Geometry check sheet. Reference: the model listing, model coordinates, mm. Coordinates: 2 decimals unless noted, no trailing zeros. Order: outer loops, then holes, each group sorted by start corner. A loop starts at its lowest first (then second) coordinate and runs counter-clockwise, first axis right, second up. Notation, with made-up numbers: (35.25, -34) -> (56.25, -34) arc R20 ccw to (56.25, -26) -> close; hole circle Ø7 at (20, 10.5). An arc over 180 degrees is marked (long way). Answer in a Markdown table with one row per item. Add a question column.
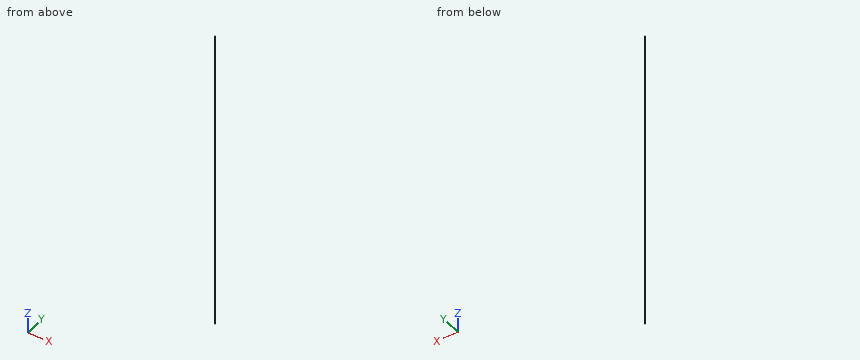
```python
from build123d import *

# Parameters (mm, degrees)
F0_R     = 4.7625
F1_DEPTH = 1295.4
F2_R     = 4.699
F3_DEPTH = 50.8
F5_SIZE  = 0.762


with BuildPart() as f1:
    # F0 (on Top) → F1 (new body, symmetric)
    with BuildSketch(Plane.XY):
        Circle(F0_R)
    extrude(amount=F1_DEPTH, both=True)

    # F2 (on face) → F3 (join)
    with BuildSketch(Plane.XY.offset(1295.4)):
        Circle(F2_R)
    extrude(amount=F3_DEPTH)

    # F4: F1 across plane


with BuildPart() as f1_1:
    add(f1.part)
    add(f1.part.mirror(Plane.XY))

    # F5
    f5_edges = [f1_1.edges().sort_by_distance(p)[0] for p in [
        (-4.699, 0, 1346.2),
        (-4.699, 0, -1346.2),
    ]]
    chamfer(f5_edges, length=F5_SIZE)


solid = f1_1.part
```
(1) Cross-section at A-A (z = 703). Enter the section's corners in (x, y) (1 decimal), plus the area to 3 significant figures.
(2) Go/stop test with flat-tipped pins: P1, Ø1, axis at y = -1, z = 203.5, coming from the +X side; P2, Ø5, axis at y = -1.5, z = 83, coming from the +X side; P3, Ø1.5, axis at x = -3.5, z = -978.5, coming from the +Y side; P4, Ø5, axis at y = -4, z = 15, coming from the +X side. Record where each tip stops, or that it passes through.
(3) Scan lines: line 1 along Y through (x, z) = (0.5, -700.5); line 2 along Y through (x, z) = (2.5, 219.5). Record each from-to range of solid material in increasing order.
Checks:
| question | item | result |
|---|---|---|
| 1 | outline | circle Ø9.5 at (0, 0) |
| 1 | area | 71.3 mm² |
| 2 | P1 | x = 4.74 |
| 2 | P2 | x = 4.76 |
| 2 | P3 | y = 3.89 |
| 2 | P4 | x = 4.52 |
| 3 | line 1 | -4.74 to 4.74 |
| 3 | line 2 | -4.05 to 4.05 |
